```python
from build123d import *

# Parameters (mm, degrees)
SKETCH1_W                       = 919.1625
SKETCH1_H                       = 463.55
BOSS_EXTRUDE1_DEPTH             = 430.2125
SHELL1_T                        = -6.35
BOSS_EXTRUDE2_REACH             = 393.414
SKETCH2_W                       = 906.4625
SKETCH2_H                       = 6.35
BOSS_EXTRUDE2_DIRECTION_2_DEPTH = 30.48


with BuildPart() as part:
    # Sketch1 → Boss-Extrude1 (new body)
    with BuildSketch(Plane(origin=(0, 0, 0), x_dir=(1, 0, 0), z_dir=(0, 1, 0))):
        with Locations((459.58125, 231.775)):
            Rectangle(SKETCH1_W, SKETCH1_H)
    extrude(amount=BOSS_EXTRUDE1_DEPTH)

    # Shell1
    shell1_openings = [part.faces().sort_by_distance(p)[0] for p in [
        (459.58125, 430.2125, -231.775),
    ]]
    offset(amount=SHELL1_T, openings=shell1_openings, kind=Kind.INTERSECTION)

    # Sketch2 → Boss-Extrude2 (add, up to next)
    with BuildSketch(Plane(origin=(0, 391.414, 0), x_dir=(1, 0, 0), z_dir=(0, 1, 0)), mode=Mode.PRIVATE) as boss_extrude2_sk1:
        with Locations((459.58125, 344.4875)):
            Rectangle(SKETCH2_W, SKETCH2_H)
    boss_extrude2_tool1 = extrude(boss_extrude2_sk1.sketch, amount=-BOSS_EXTRUDE2_REACH, mode=Mode.PRIVATE) - part.part
    add(boss_extrude2_tool1.solids().sort_by_distance((459.58125, 391.414, -344.4875))[0])
    # Sketch2 → Boss-Extrude2 (add, up to next)
    with BuildSketch(Plane(origin=(0, 391.414, 0), x_dir=(1, 0, 0), z_dir=(0, 1, 0)), mode=Mode.PRIVATE) as boss_extrude2_sk2:
        with Locations((459.58125, 228.6)):
            Rectangle(SKETCH2_W, SKETCH2_H)
    boss_extrude2_tool2 = extrude(boss_extrude2_sk2.sketch, amount=-BOSS_EXTRUDE2_REACH, mode=Mode.PRIVATE) - part.part
    add(boss_extrude2_tool2.solids().sort_by_distance((459.58125, 391.414, -228.6))[0])
    # Sketch2 → Boss-Extrude2 (add, up to next)
    with BuildSketch(Plane(origin=(0, 391.414, 0), x_dir=(1, 0, 0), z_dir=(0, 1, 0)), mode=Mode.PRIVATE) as boss_extrude2_sk3:
        with Locations((459.58125, 112.7125)):
            Rectangle(SKETCH2_W, SKETCH2_H)
    boss_extrude2_tool3 = extrude(boss_extrude2_sk3.sketch, amount=-BOSS_EXTRUDE2_REACH, mode=Mode.PRIVATE) - part.part
    add(boss_extrude2_tool3.solids().sort_by_distance((459.58125, 391.414, -112.7125))[0])

    # Sketch2 → Boss-Extrude2 direction 2 (add)
    with BuildSketch(Plane(origin=(0, 391.414, 0), x_dir=(1, 0, 0), z_dir=(0, 1, 0))):
        with Locations((459.58125, 344.4875)):
            Rectangle(SKETCH2_W, SKETCH2_H)
        with Locations((459.58125, 228.6)):
            Rectangle(SKETCH2_W, SKETCH2_H)
        with Locations((459.58125, 112.7125)):
            Rectangle(SKETCH2_W, SKETCH2_H)
    extrude(amount=BOSS_EXTRUDE2_DIRECTION_2_DEPTH)


solid = part.part
```
The listing builds one solid part. Answer for the finished solid, in the listing's coordinates (mm). A direction names the side the tool comes from. Give positions to 0.01 mm unless a question says otherwise; leave off trailing zeros. Write each loop counter-clockwise with the first axis right and the second up, starting at its lowest first coordinate (ties: lowest second). Pieces come first, ordered by that corner, then holes. Notation, with made-up numbers: (2, -4) -> (32, -4) arc R5 cw to (32, 4) -> close; hole circle Ø3 at (72, 32.5). An arc over 180 degrees is marked (long way). Use one line per item in the form item = value.
1) Section A-A on y = 75.5 is taken. Count the separate pieces of the cut face and the enclosed holes in it, plus the area to 3 significant figures.
Result:
separate_pieces = 1
enclosed_holes = 4
area = 34,700 mm²
2) Section C-C on z = -435 is taken. Write down the section's boundary in (x, y), plus the area to 3 significant figures.
Result:
outline = (0, 0) -> (919.16, 0) -> (919.16, 430.21) -> (912.81, 430.21) -> (912.81, 6.35) -> (6.35, 6.35) -> (6.35, 430.21) -> (0, 430.21) -> close
area = 11,200 mm²
3) Straight lines are drawn through the part: probe 1 along X at (y, z) = (41.5, -48); probe 2 along Y at (x, z) = (710, -192); probe 3 along Y at (x, z) = (583.5, -110.5). For each, find the intervals that lie inside material, in ascending order.
Result:
probe_1 = 0 to 6.35, 912.81 to 919.16
probe_2 = 0 to 6.35
probe_3 = 0 to 421.89
4) A tool of negligible diameter and unlimited length cuts with its end or side. For faces 1 (the flat face through (912.812, 215, -179)), 2 (the flat face through (453, 212, -463.55)), from which of +Z, -Z, +X, -X, +Y, -Y can it reach the whole face along a straight path? Write none if from no direction.
Result:
face_1 = +Y
face_2 = -Z, +X, -X, +Y, -Y
5) Each of these flat-tipped pins is pushed along its axis until it touches: P1, Ø2, axis at x = 585, z = -274, coming from the +Y side; P2, Ø5, axis at x = 438, z = -111.5, coming from the +Y side. Where does it stop, or does it pass through?
Result:
P1 = 6.35
P2 = 421.89
6) For a pull along Z with two mould halves and no side action, classify faces 3 (the flat face through (453, 212, 0)), 4 (the flat face through (453, 6.35, -287)), 5 (the flat face through (0, 212, -229)) as +Z half, -Z half, draft (parallel to the pull), parting line (faces both ways), or undercut.
Result:
face_3 = +Z half
face_4 = undercut
face_5 = draft
